from build123d import *

# Parameters (mm, degrees)
EXTRUDE_1_DEPTH     = 2
SKETCH_3_R          = 1.65
SKETCH_3_R_2        = 1.5
CUT_EXTRUDE_2_DEPTH = 10.552486587
FILLET_1_R          = 0.5


with BuildPart() as part:
    # 草图1 → 凸台-拉伸1 (new body)
    with BuildSketch(Plane(origin=(0, 0, 0), x_dir=(1, 0, 0), z_dir=(0, 1, 0))):
        with BuildLine():
            Line((-7, 2.5), (7, 2.5))
            ThreePointArc((7, 2.5), (8.414213562, 1.914213562), (9, 0.5))
            Line((9, 0.5), (9, -0.5))
            ThreePointArc((9, -0.5), (8.414213562, -1.914213562), (7, -2.5))
            Line((7, -2.5), (-7, -2.5))
            ThreePointArc((-7, -2.5), (-8.414213562, -1.914213562), (-9, -0.5))
            Line((-9, -0.5), (-9, 0.5))
            ThreePointArc((-9, 0.5), (-8.414213562, 1.914213562), (-7, 2.5))
        make_face()
    extrude(amount=EXTRUDE_1_DEPTH)

    # 草图3 → 切除-拉伸2 (cut, through all)
    with BuildSketch(Plane(origin=(0, 2, 0), x_dir=(1, 0, 0), z_dir=(0, 1, 0))):
        with Locations(Location((-5, 0, 0), (0, 0, 270))):
            Circle(SKETCH_3_R)
        with Locations(Location((5, 0, 0), (0, 0, 270))):
            Circle(SKETCH_3_R_2)
    extrude(amount=-CUT_EXTRUDE_2_DEPTH, mode=Mode.SUBTRACT)

    # 圆角1
    fillet_1_edges = [part.edges().sort_by_distance(p)[0] for p in [
        (-9, 0, 0),
        (-8.414213562, 0, -1.914213562),
        (0, 0, -2.5),
        (8.414213562, 0, -1.914213562),
        (-8.414213562, 2, -1.914213562),
        (-9, 2, 0),
        (-8.414213562, 2, 1.914213562),
        (0, 2, 2.5),
        (8.414213562, 2, 1.914213562),
        (9, 2, 0),
        (8.414213562, 2, -1.914213562),
        (9, 0, 0),
        (0, 2, -2.5),
        (8.414213562, 0, 1.914213562),
        (0, 0, 2.5),
        (-8.414213562, 0, 1.914213562),
    ]]
    fillet(fillet_1_edges, radius=FILLET_1_R)


solid = part.part
Geometry: final body of the model. Coordinates: model frame, mm. Coordinates: 2 decimals unless noted, no trailing zeros. Write each loop counter-clockwise with the first axis right and the second up, starting at its lowest first coordinate (ties: lowest second). Pieces come first, ordered by that corner, then holes. Notation, with made-up numbers: (39, -20) - (88, -20) arc R21 ccw to (88, 5) - close; hole circle Ø10 at (-32, 51). An arc over 180 degrees is marked (long way). Return JSON: item names as keys, results as strings.
Item 1: Section query D-D (x = -0.5). Output: boundary loops of the cut face in (y, z).
Completed:
{"outline": "(0, -2) arc R0.5 ccw to (0.5, -2.5) - (1.5, -2.5) arc R0.5 ccw to (2, -2) - (2, 2) arc R0.5 ccw to (1.5, 2.5) - (0.5, 2.5) arc R0.5 ccw to (0, 2) - close"}
Item 2: Pull-direction query (X, two-part tool) for faces 1 (the face through (9, 1, 0)), 2 (the face through (0, 0, 0)), 3 (the face through (-6.6, 1, -0.4)); classes: +X half, -X half, draft (parallel to the pull), parting line (faces both ways), or undercut.
Completed:
{"face 1": "+X half", "face 2": "draft", "face 3": "undercut"}
Item 3: Line query: L1, parallel to X at y = 1.8, z = -0.95; L2, parallel to X at y = 1.55, z = -0.55; L3, parallel to Z at x = 4.5, y = 0.35. Output: solid intervals per line, ascending.
Completed:
{"L1": "x = -8.85 to -6.35, -3.65 to 3.84, 6.16 to 8.85", "L2": "x = -9 to -6.56, -3.44 to 3.6, 6.4 to 9", "L3": "z = -2.48 to -1.41, 1.41 to 2.48"}
Item 4: Pin query (flat end, axial travel): pin 1 Ø2 at (x, z) = (-5, 0) entering from +Y. Return the tip coordinate at first contact, or that it passes through.
Completed:
{"pin 1": "passes through"}
Item 5: Section query A-A (x = -5). Output: boundary loops of the cut face in (y, z), and give its area (3 significant figures).
Completed:
{"outline": "(0, -2) arc R0.5 ccw to (0.5, -2.5) - (1.5, -2.5) arc R0.5 ccw to (2, -2) - (2, -1.65) - (0, -1.65) - close; (0, 1.65) - (2, 1.65) - (2, 2) arc R0.5 ccw to (1.5, 2.5) - (0.5, 2.5) arc R0.5 ccw to (0, 2) - close", "area": "3.19 mm2"}
Item 6: Section query C-C (z = 0). Output: boundary loops of the cut face in (x, y).
Completed:
{"outline": "(-9, 0.5) arc R0.5 ccw to (-8.5, 0) - (-6.65, 0) - (-6.65, 2) - (-8.5, 2) arc R0.5 ccw to (-9, 1.5) - close; (-3.35, 0) - (3.5, 0) - (3.5, 2) - (-3.35, 2) - close; (6.5, 0) - (8.5, 0) arc R0.5 ccw to (9, 0.5) - (9, 1.5) arc R0.5 ccw to (8.5, 2) - (6.5, 2) - close"}
Item 7: Section query B-B (y = 1.8). Output: boundary loops of the cut face in (x, z), and give its area (3 significant figures).
Completed:
{"outline": "(-8.9, -0.5) arc R1.9 ccw to (-7, -2.4) - (7, -2.4) arc R1.9 ccw to (8.9, -0.5) - (8.9, 0.5) arc R1.9 ccw to (7, 2.4) - (-7, 2.4) arc R1.9 ccw to (-8.9, 0.5) - close; hole circle Ø3.3 at (-5, 0); hole circle Ø3 at (5, 0)", "area": "66.7 mm2"}
